Read the model definition and answer for the solid it produces. Units are mm, in the model's axes. Coordinates: 2 decimals unless noted, no trailing zeros. Loops run counter-clockwise (first coordinate to the right, second up) from the corner with the lowest first, then second, coordinate; pieces in that order, holes last. Notation, with made-up numbers: (18, -5) -> (53, -5) arc R21 ccw to (53, 16) -> close; hole circle Ø1 at (-29, 28.25). An arc over 180 degrees is marked (long way). Answer as a JSON object with one key per item and string values. Group by question number.
1) Flat-ended cylindrical pins translate along their axes: P1, Ø2, axis at x = 37, y = 37, coming from the +Z side; P2, Ø2.5, axis at x = 0, y = -7, coming from the -Z side; P3, Ø5, axis at y = 21, z = 15, coming from the +X side; P4, Ø3, axis at x = 0, y = 7, coming from the +Z side. Find the tip coordinate at first contact, or state that the pin passes through.
2) Determine the mould class of faces 1 (the face through (38.24, 37.39, 19.53)), 2 (the face through (11.923, 3.755, 10.916)) for opening direction X: released by +X, released by -X, zero draft, split by the parting line, or undercut.
3) Section C-C, the plane z = 13.25 is taken. Count the separate pieces of the cut face and the enclosed holes in it, plus the area to 3 significant figures.
4) Section A-A, the plane x = 30.5 is taken. Give the vertices of the cut face in (y, z).
5) Consider probe 1 along X at (y, z) = (37.5, 18.75); probe 2 along X at (y, z) = (36, 18.75); probe 3 along Z at (x, y) = (-16.5, -38). Determine where each line is inside the solid, lowest interval first. Write a range as [from, to].
from build123d import *

# Parameters (mm, degrees)
SKETCH003_R     = 12.5
SKETCH003_R_2   = 1.3
PAD_DEPTH       = 12
PAD001_DEPTH    = 0.8
SKETCH005_W     = 84
SKETCH005_H     = 84
PAD002_DEPTH    = 5
SKETCH030_R     = 1.3
POCKET014_DEPTH = 17.8034874046


with BuildPart() as part:
    # Sketch003 (on DatumPlane) → Pad (new body)
    with BuildSketch(Plane(origin=(0.0002244487, 4.55156e-05, 5.000457982), x_dir=(0.999999999, -4e-10, -4.48856e-05), z_dir=(4.48856e-05, 9.1023e-06, 0.999999999))):
        Circle(SKETCH003_R)
        with Locations((0, 7)):
            Circle(SKETCH003_R_2, mode=Mode.SUBTRACT)
        with Locations((0, -7)):
            Circle(SKETCH003_R_2, mode=Mode.SUBTRACT)
    extrude(amount=PAD_DEPTH)

    # Sketch004 (on Face1 of CopyPocket002) → Pad001 (join)
    with BuildSketch(Plane(origin=(0.0002244487, 4.55156e-05, 5.000457982), x_dir=(0.999999999, -4e-10, -4.48856e-05), z_dir=(4.48856e-05, 9.1023e-06, 0.999999999))):
        Polygon((4.9, 0), (-2.45, 4.2435244785), (-2.45, -4.2435244785), align=None)
    extrude(amount=-PAD001_DEPTH)

    # Sketch005 (on Face3 of Pad001) → Pad002 (join)
    with BuildSketch(Plane(origin=(0.0007630761, 0.000154743, 17.0004579694), x_dir=(0.999999999, -4e-10, -4.48856e-05), z_dir=(4.48856e-05, 9.1023e-06, 0.999999999))):
        Rectangle(SKETCH005_W, SKETCH005_H)
    extrude(amount=PAD002_DEPTH)

    # Sketch030 (on Face5 of Pad002) → Pocket014 (cut, through all)
    with BuildSketch(Plane(origin=(0.0009875042, 0.0002002544, 22.0004579641), x_dir=(0.999999999, -4e-10, -4.48856e-05), z_dir=(4.48856e-05, 9.1023e-06, 0.999999999))):
        with Locations((-37, 37)):
            Circle(SKETCH030_R)
        with Locations((-37, -37)):
            Circle(SKETCH030_R)
        with Locations((37, -37)):
            Circle(SKETCH030_R)
        with Locations((37, 37)):
            Circle(SKETCH030_R)
    extrude(amount=-POCKET014_DEPTH, mode=Mode.SUBTRACT)


solid = part.part
Determined:
{
 "1": {"P1": "through", "P2": "z = 17", "P3": "x = 42", "P4": "z = 22"},
 "2": {"face 1": "undercut", "face 2": "split by the parting line"},
 "3": {"separate pieces": "1", "enclosed holes": "2", "area": "480 mm²"},
 "4": {"outline": "(-42, 17) -> (42, 17) -> (42, 22) -> (-42, 22) -> close"},
 "5": {"probe 1": "[-42, -38.2], [-35.8, 35.8], [38.2, 42]", "probe 2": "[-42, -37.83], [-36.17, 36.17], [37.83, 42]", "probe 3": "[17, 22]"}
}
